Can you work these out from the model? Positions are in its coordinate system, mm. A direction names the side the tool comes from. Round coordinates to 2 decimals unless told otherwise and drop trailing zeros. Loops run counter-clockwise (first coordinate to the right, second up) from the corner with the lowest first, then second, coordinate; pieces in that order, holes last. Notation, with made-up numbers: (-11, -1.75) - (26, -1.75) arc R27 ccw to (26, 26.25) - close; hole circle Ø9 at (-35.75, 40). An arc over 180 degrees is marked (long way). Answer as CSV lines item,"result".
Autodesk Inventor part; units mm, degrees
ref_plane "Work Plane1" through (13.5, 0, 0) normal (1, 0, 0) x (0, 0, -1)
ref_plane "YZ Plane" through (0, 0, 0) normal (1, 0, 0) x (0, 1, 0)
ref_plane "XZ Plane" through (0, 0, 0) normal (0, 1, 0) x (-1, 0, 0)
sketch "Sketch1" plane through (0, 0, 0) normal (1, 0, 0) x (0, 1, 0)
  circle A0 centre (0, 0) radius 1.5
  dimension "d0" = 3
extrude "Extrusion1" add sketch "Sketch1" along normal blind 8
sketch "Sketch2" plane through (8, 0, 0) normal (1, 0, 0) x (0, 0, -1)
  circle A0 centre (0, 0) radius 2.25
  dimension "d3" = 4.5
extrude "Extrusion2" add sketch "Sketch2" along normal blind 3
ref_plane "Work Plane1" through (13.5, 0, 0) normal (1, 0, 0) x (0, 0, -1)
fillet "Fillet2" radius 0.2 1 edges at (11, 0, 2.25)
sketch "Sketch4" plane through (11, 0, 0) normal (1, 0, 0) x (0, 0, -1)
  line L0 (1.2, 0) -> (0.6, -1.0392)
  line L1 (0.6, -1.0392) -> (-0.6, -1.0392)
  line L2 (-0.6, -1.0392) -> (-1.2, 0)
  line L3 (-1.2, 0) -> (-0.6, 1.0392)
  line L4 (-0.6, 1.0392) -> (0.6, 1.0392)
  line L5 (0.6, 1.0392) -> (1.2, 0)
  point P0 (0, 0)
  point P1 (0, 0)
  dimension "d14" = 2.4
  dimension "d15" = 1.0392
extrude "Extrusion4" cut sketch "Sketch4" against normal blind 1.5
properties part number "M3" material "Iron, Cast"
Q1. We'd pull the mould along Z, two halves only. Please class faces 1 (the flat face through (0, 0, 0)), 2 (the flat face through (10.26, 0.527, -0.896)), 3 (the cylindrical face through (9.38, -2.23, 0.29)): pulls with the +Z half, pulls with the -Z half, needs draft (parallel to the pull), parting line crosses it, or undercut.
Checks:
face 1,"needs draft"
face 2,"undercut"
face 3,"parting line crosses it"
Q2. On a 3-axis mill with a long thin cutter (end or side, diameter ignored), from which of +Z, -Z, +X, -X, +Y, -Y can I reach the whole of each face in a straight line? I mean faces 4 (the flat face through (11, -1, -1)), 5 (the flat face through (10.26, -0.512, -0.904)), 6 (the cylindrical face through (3.94, -1.5, -0.07)). Say none if no direction works.
Checks:
face 4,"+Z, -Z, +X, +Y, -Y"
face 5,"+X"
face 6,"-X"
Q3. Imagine slicing it at C-C (x = 9). Write out the boundary of the cut face in (y, z), then the cut area to 3 significant figures.
Checks:
outline,"circle Ø4.5 at (0, 0)"
area,"15.9 mm²"
Q4. Imagine slicing it at A-A (z = 0). Write out the boundary of the cut face in (x, y), then the cut area to 3 significant figures.
Checks:
outline,"(0, -1.5) - (8, -1.5) - (8, -2.25) - (10.8, -2.25) arc R0.2 ccw to (11, -2.05) - (11, -1.04) - (9.5, -1.04) - (9.5, 1.04) - (11, 1.04) - (11, 2.05) arc R0.2 ccw to (10.8, 2.25) - (8, 2.25) - (8, 1.5) - (0, 1.5) - close"
area,"34.4 mm²"
Q5. Imagine slicing it at B-B (x = 2.5). Write out the boundary of the cut face in (y, z).
Checks:
outline,"circle Ø3 at (0, 0)"
Q6. If I drill on line 1 along X through (y, z) = (0.25, -0.2); line 2 along X through (y, z) = (1.9, -0.1); line 3 along Y through (x, z) = (9.75, 0.3), over which ranges is the centre line in solid material (lowest first)? Write a range as [from, to].
Checks:
line 1,"[0, 9.5]"
line 2,"[8, 11]"
line 3,"[-2.23, -1.04], [1.04, 2.23]"
Q7. I'm going to push flat-ended pins straight in: pin 1 Ø2 at (y, z) = (-0.5, -0.5) entering from -X; pin 2 Ø1 at (y, z) = (-0.5, 0) entering from +X; pin 3 Ø1 at (x, z) = (8.5, 1) entering from +Y. Where does each tip first touch, or does it pass through?
Checks:
pin 1,"x = 0"
pin 2,"x = 9.5"
pin 3,"y = 2.19"
